Source: CAD feature listing. Evaluate the final solid. Frame: model axes, mm. Face numbers are marked on the shaded views. A direction names the side the tool comes from. Give positions to 0.01 mm unless a question says otherwise; leave off trailing zeros. Write each loop counter-clockwise with the first axis right and the second up, starting at its lowest first coordinate (ties: lowest second). Pieces come first, ordered by that corner, then holes. Notation, with made-up numbers: (70.5, 41.25) -> (89.5, 41.25) arc R14 ccw to (89.5, 51.25) -> close; hole circle Ø3 at (-1.75, 74.25). An arc over 180 degrees is marked (long way). Answer as a JSON object with one key per item and string values. Group by question number.
Item 1: Section query C-C on z = 132.5. Return the cut outline in (x, y).
Item 2: Section query A-A on y = 0. Return the cut outline in (x, z).
Item 3: First-contact query: pin 1 Ø5 at (y, z) = (0, 132.5) entering from -X; pin 2 Ø22.5 at (x, y) = (36.5, 7.5) entering from +Z; pin 3 Ø15 at (y, z) = (-5, 52.5) entering from -X; pin 4 Ø12 at (y, z) = (0.5, 55.5) entering from +X. Flat tips, straight axial feed; report the tip coordinate or a pass-through.
Item 4: Section query B-B on x = 50. Return the cut outline in (y, z), plus the area to 3 significant figures.
Item 5: Access query for the marked faces 1, 2, 3 and 4. Directions: +Z, -Z, +X, -X, +Y, -Y. A direction counts if a zero-diameter tool reaches every point of the face in a straight line with its end or side. Return the directions, or none.
Item 6: Ray query, probe 1 along Z at (x, y) = (-50, -1); probe 2 along Z at (x, y) = (18, -11.5); probe 3 along Y at (x, z) = (69, 132.5). Return the intervals inside material, ascending. Write a range as from..to.
Item 7: Pull-direction query (Z, two-part tool) for the marked faces 5, 6 and 7; classes: pulls with the +Z half, pulls with the -Z half, needs draft (parallel to the pull), parting line crosses it, or undercut.
Item 8: Section query D-D on x = -23. Return the cut outline in (y, z).
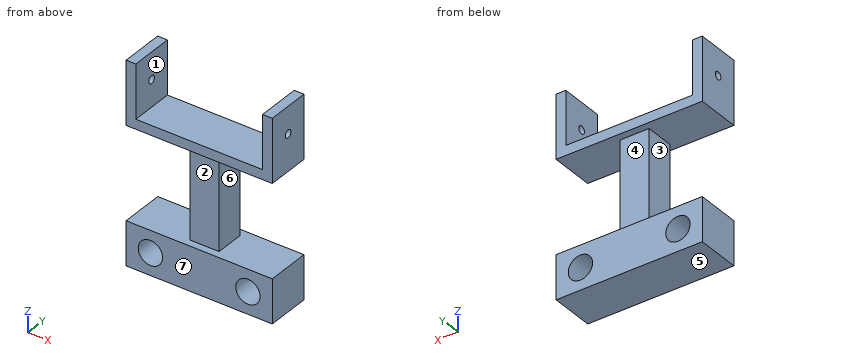
from build123d import *

# Parameters (mm, degrees)
SKETCH_1_W               = 150
SKETCH_1_H               = 45
EXTRUDE_1_DEPTH          = 45
CUT_EXTRUDE_1_DEPTH      = 91.311959341
CUT_EXTRUDE_1_DEPTH_BACK = 91.311959341
SKETCH_2_R               = 12.5
SKETCH_3_W               = 30
SKETCH_3_H               = 30
EXTRUDE_2_DEPTH          = 95
EXTRUDE_3_DEPTH          = 22.5
CUT_EXTRUDE_2_DEPTH      = 179.132675273
CUT_EXTRUDE_2_DEPTH_BACK = 179.132675273
SKETCH_5_R               = 4


with BuildPart() as part:
    # 草图1 → 凸台-拉伸1 (new body)
    with BuildSketch(Plane.XY):
        Rectangle(SKETCH_1_W, SKETCH_1_H)
    extrude(amount=-EXTRUDE_1_DEPTH)

    # 草图2 → 切除-拉伸1 (cut, two sides: drawn at the far end of the back side and taken through both)
    with BuildSketch(Plane(origin=(0, 0, 0), x_dir=(1, 0, 0), z_dir=(0, 1, 0)).offset(-CUT_EXTRUDE_1_DEPTH_BACK)):
        with Locations(Location((-50, 22.5, 0), (0, 0, 270))):
            Circle(SKETCH_2_R)
        with Locations(Location((50, 22.5, 0), (0, 0, 270))):
            Circle(SKETCH_2_R)
    extrude(amount=CUT_EXTRUDE_1_DEPTH + CUT_EXTRUDE_1_DEPTH_BACK, mode=Mode.SUBTRACT)

    # 草图3 → 凸台-拉伸2 (add)
    with BuildSketch(Plane.XY):
        Rectangle(SKETCH_3_W, SKETCH_3_H)
    extrude(amount=EXTRUDE_2_DEPTH)

    # 草图4 → 凸台-拉伸3 (add, symmetric)
    with BuildSketch(Plane(origin=(0, 0, 0), x_dir=(1, 0, 0), z_dir=(0, 1, 0))):
        Polygon((-75, -95), (75, -95), (75, -160), (65, -160), (65, -105), (-65, -105), (-65, -160), (-75, -160), align=None)
    extrude(amount=EXTRUDE_3_DEPTH, both=True)

    # 草图5 → 切除-拉伸2 (cut, two sides: drawn at the far end of the back side and taken through both)
    with BuildSketch(Plane(origin=(0, 0, 0), x_dir=(0, 0, -1), z_dir=(1, 0, 0)).offset(-CUT_EXTRUDE_2_DEPTH_BACK)):
        with Locations((-132.5, 0)):
            Circle(SKETCH_5_R)
    extrude(amount=CUT_EXTRUDE_2_DEPTH + CUT_EXTRUDE_2_DEPTH_BACK, mode=Mode.SUBTRACT)


solid = part.part
Worked answers:
{
 "1": {"outline": "(-75, -22.5) -> (-65, -22.5) -> (-65, -4) -> (-75, -4) -> close; (-75, 4) -> (-65, 4) -> (-65, 22.5) -> (-75, 22.5) -> close; (65, -22.5) -> (75, -22.5) -> (75, -4) -> (65, -4) -> close; (65, 4) -> (75, 4) -> (75, 22.5) -> (65, 22.5) -> close"},
 "2": {"outline": "(-75, -45) -> (75, -45) -> (75, 0) -> (15, 0) -> (15, 95) -> (75, 95) -> (75, 128.5) -> (65, 128.5) -> (65, 105) -> (-65, 105) -> (-65, 128.5) -> (-75, 128.5) -> (-75, 95) -> (-15, 95) -> (-15, 0) -> (-75, 0) -> close; (-75, 136.5) -> (-65, 136.5) -> (-65, 160) -> (-75, 160) -> close; (65, 136.5) -> (75, 136.5) -> (75, 160) -> (65, 160) -> close; hole circle Ø25 at (-50, -22.5); hole circle Ø25 at (50, -22.5)"},
 "3": {"pin 1": "through", "pin 2": "z = 105", "pin 3": "x = -15", "pin 4": "x = 15"},
 "4": {"outline": "(-22.5, -45) -> (22.5, -45) -> (22.5, -35) -> (-22.5, -35) -> close; (-22.5, -10) -> (22.5, -10) -> (22.5, 0) -> (-22.5, 0) -> close; (-22.5, 95) -> (22.5, 95) -> (22.5, 105) -> (-22.5, 105) -> close", "area": "1,350 mm^2"},
 "5": {"face 1": "+Z, +Y, -Y", "face 2": "+X, -X, -Y", "face 3": "-X, +Y, -Y", "face 4": "+X, -X, +Y"},
 "6": {"probe 1": "-45..-35, -10..0, 95..105", "probe 2": "-45..0, 95..105", "probe 3": "-22.5..-4, 4..22.5"},
 "7": {"face 5": "pulls with the -Z half", "face 6": "undercut", "face 7": "needs draft"},
 "8": {"outline": "(-22.5, -45) -> (22.5, -45) -> (22.5, 0) -> (-22.5, 0) -> close; (-22.5, 95) -> (22.5, 95) -> (22.5, 105) -> (-22.5, 105) -> close"}
}
